For this review, take the finished solid that the model builds, in its own axes (mm). A direction names the side the tool comes from. Coordinates: 2 decimals unless noted, no trailing zeros. Order: outer loops, then holes, each group sorted by start corner. A loop starts at its lowest first (then second) coordinate and runs counter-clockwise, first axis right, second up. Notation, with made-up numbers: (-11, 35.25) -> (29, 35.25) arc R22 cw to (29, 49.25) -> close; hole circle Ø9 at (16.25, -39.5). An arc over 180 degrees is marked (long way). Return JSON: item names as keys, results as strings. Group by question number.
Item 1: Take a section at B-B (x = -5). Write out the cut boundary in (y, z), then the cut area to 3 significant figures.
Item 2: Take a section at A-A (z = 15.5). Write out the cut boundary in (x, y).
Item 3: Machinability: for faces 1 (the flat face through (50, 2, -67)), 2 (the flat face through (70, 4, 13.5)), 3 (the flat face through (13.7, 5, -126.3)), which of the approach directions +Z, -Z, +X, -X, +Y, -Y give a long, thin tool a straight path to every point of the face, cutting with its end or side? Answer none if there is none.
Item 4: Take a section at C-C (y = 1.75). Count the separate pieces of the cut face and the enclosed holes in it, then the cut area to 3 significant figures.
Item 5: Insertion check: pin 1 (1 mm diameter, centred on x = 22, y = 1.5, fed in from +Z); pin 2 (3 mm diameter, centred on x = 15.5, z = -20.5, fed in from +Y); pin 3 (1.6 mm diameter, centred on x = 28, y = 4, fed in from -Z). Each pin has a flat end and moves straight along its axis. Give the tip position at first contact, or say it passes through.
Item 6: Draft analysis for pull direction Z (two halves, no side actions). For faces 4 (the flat face through (-11, 4, 0)), 5 (the flat face through (-10.5, 4, 4)), 6 (the flat face through (-23.5, 4, 22)), 7 (the flat face through (0, 2, -68)), state which applies: +Z half, -Z half, draft (parallel to the pull), parting line (faces both ways), or undercut.
Item 7: For line 1 along X through (y, z) = (1.3, -125); line 2 along X through (y, z) = (5, 4); line 3 along X through (y, z) = (2.5, -60), list the stretches that pass through material, from the lowest coordinate up.
Item 8: Take a section at D-D (x = -19). Write out the cut boundary in (y, z).
Autodesk Inventor part; units mm, degrees
ref_plane "Płaszczyzna konstrukcyjna1" through (25, 3, -61.25) normal (1, 0, 0) x (0, 0, 1)
ref_plane "YZ Plane" through (0, 0, 0) normal (1, 0, 0) x (0, 1, 0)
ref_plane "XZ Plane" through (0, 0, 0) normal (0, 1, 0) x (-1, 0, 0)
sketch "Szkic1" plane through (0, 0, 0) normal (0, 1, 0) x (-1, 0, 0)
  line L0 (0, 0) -> (-25, 0)
  line L1 (-25, 0) -> (-25, -135)
  line L2 (-25, -135) -> (0, -135)
  line L3 (0, -135) -> (0, 0)
  line L4 (-5, -2) -> (-25, -2)
  line L5 (-25, -2) -> (-25, -115)
  line L6 (-25, -115) -> (-5, -115)
  line L7 (-5, -115) -> (-5, -2)
  line L8 (-25, -115) -> (-5, -2)
  line L9 (-20, -115) -> (-5, -30.25)
  line L10 (-5, -30.25) -> (-5, -2)
  line L11 (-25, -115) -> (-20, -115)
  dimension "d0" = 25
  dimension "d1" = 135
  dimension "d2" = 5
  dimension "d3" = 20
  dimension "d4" = 2
  dimension "d7" = 5
extrude "Wyciągnięcie proste2" add sketch "Szkic1" along normal blind 5 contours L3 L2 L1 L6 L7 L4 L0 | L8 L7 L9 L6
sketch "Szkic2" plane through (25, 0, 0) normal (1, 0, 0) x (0, 0, -1)
  line L0 (0, 0) -> (-33, 0)
  line L1 (-33, 0) -> (-33, 7)
  line L2 (-33, 7) -> (0, 7)
  line L3 (0, 7) -> (0, 0)
  line L4 (-33, 0) -> (-30, 7)
  dimension "d10" = 33
  dimension "d11" = 7
  dimension "d12" = 30
extrude "Wyciągnięcie proste3" add sketch "Szkic2" against normal blind 50 contours L0 L4 L2 L3
sketch "Szkic3" plane through (25, 7, 30) normal (0, 1, 0) x (1, 0, 0)
  line L0 (0, 0) -> (-50, 0)
  line L1 (0, 0) -> (-48.5, 0)
  line L2 (-48.5, 0) -> (-48.5, 28.5)
  line L3 (-48.5, 28.5) -> (0, 28.5)
  line L4 (-50, 0) -> (-50, 30)
  line L5 (-48.5, 28.5) -> (-41.5, 28.5)
  line L6 (-41.5, 28.5) -> (-41.5, 16.5)
  line L7 (-41.5, 16.5) -> (-48.5, 16.5)
  line L8 (-48.5, 16.5) -> (-48.5, 28.5)
  circle A0 centre (-41.5, 22.5) radius 6
  line L9 (-35.5, 22.5) -> (-41.5, 22.5)
  line L10 (-41.5, 22.5) -> (-41.5, 28.5)
  line L11 (-41.5, 28.5) -> (-35.5, 28.5)
  line L12 (-35.5, 28.5) -> (-35.5, 22.5)
  line L13 (0, 30) -> (-50, 30)
  line L14 (0, 30) -> (0, 0)
  line L15 (-19, 28.5) -> (-7, 28.5) construction
  line L16 (-22.5355, 28.5) -> (-19, 28.5)
  line L17 (-7, 28.5) -> (-5, 28.5)
  line L18 (-7, 0) -> (-5, 0)
  point P0 (-25, 30)
  dimension "d16" = 1.5
  dimension "d19" = 13
  dimension "d20" = 12
  dimension "d66" = 1.5
extrude "Wyciągnięcie proste4" cut sketch "Szkic3" against normal up to next contours L0 L2 L7 A0 L12 L3 L14
sketch "Szkic4" plane through (0, 5, 0) normal (0, 1, 0) x (1, 0, 0)
  line L0 (0, 0) -> (0, 17) construction
  line L1 (0, 135) -> (0, 0) construction
  line L2 (0, 17) -> (25, 17)
  line L3 (25, 17) -> (25, 24)
  line L4 (25, 24) -> (0, 24)
  line L5 (0, 24) -> (0, 17)
  dimension "d26" = 17
  dimension "d27" = 7
extrude "Wyciągnięcie proste5" add sketch "Szkic4" against normal blind 2
sketch "Szkic5" plane through (0, 5, 0) normal (0, 1, 0) x (1, 0, 0)
  line L0 (25, 115) -> (25, 135)
  line L1 (0, 135) -> (0, 0)
  line L2 (25, 135) -> (0, 135)
  line L3 (0, 135) -> (0, 110)
  line L4 (0, 110) -> (25, 110)
  line L5 (25, 110) -> (25, 135)
  circle A0 centre (15, 125) radius 3
  dimension "d30" = 25
  dimension "d31" = 6
  dimension "d32" = 10
  dimension "d33" = 10
extrude "Wyciągnięcie proste6" cut sketch "Szkic5" against normal blind 2
chamfer "Faza2" distance 2 distance2 1 1 edges at (12, 3, -125) measured on face at (17.3983, 3.6667, -123.1978)
chamfer "Faza3" distance 2 angle 45 1 edges at (12.5, 5, 0)
sketch "Szkic6" plane through (15, 5, -125) normal (0, 1, 0) x (1, 0, 0)
  point P0 (-15, -125)
  point P1 (0, 0)
hole "Otwór1" at (15, 5, -125) direction (0, -1, 0) diameter 3 end through all
sketch "Szkic7" plane through (-25, 7, 30) normal (0, 1, 0) x (1, 0, 0)
  line L0 (14.5, 28.5) -> (14.5, 22.5) construction
  line L1 (14.5, 28.5) -> (14.5, 20) construction
  line L2 (14.5, 20) -> (1.5, 20) construction
  line L3 (1.5, 16.5) -> (1.5, 0) construction
  line L4 (1.5, 20) -> (1.5, 16.5) construction
  line L5 (1.5, 20) -> (10, 20) construction
  point P0 (25, 30)
  point P1 (12.5, 27.5)
  dimension "d49" = 8.5
  dimension "d50" = 8.5
hole "Otwór2" at (-15, 7, 10) direction (0, -1, 0) diameter 3 end through all
sketch "Szkic8" plane through (0, 5, 0) normal (0, 1, 0) x (1, 0, 0)
  line L0 (25, 24) -> (25, 17) construction
  line L1 (25, 20.5) -> (15.5, 20.5) construction
  point P0 (0, 0)
  dimension "d58" = 9.5
hole "Otwór3" at (15.5, 5, -20.5) direction (0, -1, 0) diameter 2 end through all
ref_plane "Płaszczyzna konstrukcyjna1" through (25, 3, -61.25) normal (1, 0, 0) x (0, 0, 1)
mirror "Odbij1" about plane through (25, 3, -61.25) normal (1, 0, 0)
sketch "Szkic9" plane through (-25, 7, 30) normal (0, 1, 0) x (1, 0, 0)
  line L0 (14.5, 28.5) -> (85.5, 28.5)
  line L1 (27.4645, 28.5) -> (27.4645, 30)
  line L2 (72.5355, 28.5) -> (57, 12.9645)
  line L3 (72.5355, 28.5) -> (72.5355, 30)
  line L4 (75, 30) -> (25, 30)
  line L5 (27.4645, 30) -> (72.5355, 30)
  line L6 (27.4645, 28.5) -> (32.9645, 23)
  line L7 (27.4645, 28.5) -> (43, 12.9645)
  line L8 (32.9645, 23) -> (67.0355, 23)
  line L9 (85.5, 28.5) -> (14.5, 28.5)
  line L10 (72.5355, 28.5) -> (67.0355, 23)
  dimension "d71" = 7
extrude "Wyciągnięcie proste7" cut sketch "Szkic9" against normal blind 2
properties part number "lf2"
Findings below:
{
 "1": {"outline": "(0, 0) -> (7, 0) -> (7, 1.5) -> (0, 1.5) -> close; (0, 30) -> (7, 30) -> (0, 33) -> close", "area": "21.0 mm2"},
 "2": {"outline": "(-25, 0) -> (-23.5, 0) -> (-23.5, 7) -> (-25, 7) -> close; (73.5, 0) -> (75, 0) -> (75, 7) -> (73.5, 7) -> close"},
 "3": {"face 1": "-Z, +X, +Y, -Y", "face 2": "+Y, -Y", "face 3": "-Z, +X, -X, +Y"},
 "4": {"separate pieces": "1", "enclosed holes": "8", "area": "3,950 mm2"},
 "5": {"pin 1": "stops at z = 32.57", "pin 2": "stops at y = 5", "pin 3": "stops at z = -110"},
 "6": {"face 4": "-Z half", "face 5": "undercut", "face 6": "undercut", "face 7": "draft"},
 "7": {"line 1": "x = 0 to 13.5, 16.5 to 33.5, 36.5 to 50", "line 2": "x = -25 to -10.5, 60.5 to 75", "line 3": "x = 0 to 5, 10.27 to 15.27, 34.73 to 39.73, 45 to 50"},
 "8": {"outline": "(0, 0) -> (7, 0) -> (7, 13.5) -> (0, 13.5) -> close; (0, 30) -> (7, 30) -> (0, 33) -> close"}
}
